For this review, take the finished solid that the model builds, in its own axes (mm). Give positions to 0.01 mm unless a question says otherwise; leave off trailing zeros. Write each loop counter-clockwise with the first axis right and the second up, starting at its lowest first coordinate (ties: lowest second). Pieces come first, ordered by that corner, then holes. Notation, with made-up numbers: M 47,-24.75 L 62,-24.75 A33 cw 62,10.25 Z; hole C -22,80 d11. An arc over 180 degrees is marked long. Use one line per item in the form item = value. Start each with the question number.
Q1. Consider section B-B on y = 0.5. Give the number of separate pieces and of enclosed holes in the cut face, and give its area (3 significant figures).
Q2. For probe 1 along X at (y, z) = (2.25, 0); probe 2 along Z at (x, y) = (5.09, 0.45); probe 3 along X at (y, z) = (2.55, -5.5), list the stretches that pass through material, from the lowest coordinate up. Write a range as [from, to].
Q3. Consider section A-A on x = 0.01. Write out the cut boundary in (y, z), and give its area (3 significant figures).
Q4. Clearance check with flat-ended pins moving along their axes: pin 1 Ø0.5 at (x, y) = (5.5, 2) entering from +Z; pin 2 Ø0.5 at (x, y) = (3, 2) entering from -Z; pin 3 Ø0.5 at (y, z) = (2, -4) entering from -X. State where each tip first meets the part, or that it passes through.
Q5. Consider section C-C on z = 4.5. Write out the cut boundary in (x, y), and give its area (3 significant figures).
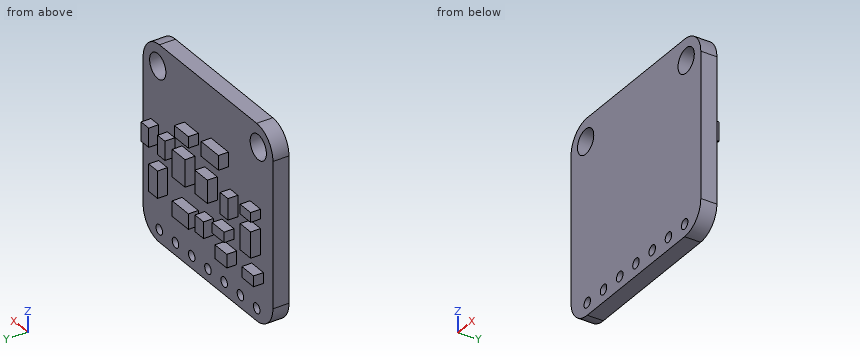
```python
from build123d import *

# Parameters (mm, degrees)
PCB_DEPTH          = 1.651
SKETCH2_R          = 1.27
SKETCH2_R_2        = 0.508
CUT_EXTRUDE1_DEPTH = 2.651
SKETCH3_W          = 1.9431
SKETCH3_H          = 2.3622
SKETCH3_W_2        = 2.0066
SKETCH3_H_2        = 2.794
SKETCH3_W_3        = 2.16822249
SKETCH3_H_3        = 1.167787324
SKETCH3_W_4        = 2.716171955
SKETCH3_H_4        = 1.493517176
SKETCH3_W_5        = 1.209663862
SKETCH3_H_5        = 2.17508788
SKETCH3_W_6        = 1.633321627
SKETCH3_H_6        = 2.659890245
SKETCH3_W_7        = 1.834361491
SKETCH3_H_7        = 1.100221283
SKETCH3_W_8        = 1.848311781
SKETCH3_H_8        = 1.38602823
SKETCH3_W_9        = 1.877433771
SKETCH3_H_9        = 1.066217503
SKETCH3_H_10       = 0.988618516
SKETCH3_W_10       = 1.152895283
SKETCH3_H_11       = 1.952725423
SKETCH3_W_11       = 1.201658639
SKETCH3_W_12       = 1.378437796
SKETCH3_H_12       = 2.778082819
SKETCH3_W_13       = 2.534678464
SKETCH3_H_13       = 1.568516227
SKETCH3_W_14       = 1.344087022
SKETCH3_H_14       = 1.688234225
COMPONENTS_DEPTH   = 1.016


with BuildPart() as part:
    # Sketch1 → pcb (new body)
    with BuildSketch(Plane(origin=(0, 0, 0), x_dir=(1, 0, 0), z_dir=(0, 1, 0))):
        with BuildLine():
            Line((-7.61, -10), (7.61, -10))
            ThreePointArc((7.61, -10), (9.406051224, -9.256051224), (10.15, -7.46))
            Line((10.15, -7.46), (10.15, 7.46))
            ThreePointArc((10.15, 7.46), (9.406051224, 9.256051224), (7.61, 10))
            Line((7.61, 10), (-7.61, 10))
            ThreePointArc((-7.61, 10), (-9.406051224, 9.256051224), (-10.15, 7.46))
            Line((-10.15, 7.46), (-10.15, -7.46))
            ThreePointArc((-10.15, -7.46), (-9.406051224, -9.256051224), (-7.61, -10))
        make_face()
    extrude(amount=PCB_DEPTH)

    # Sketch2 → Cut-Extrude1 (cut, through all)
    with BuildSketch(Plane.XZ):
        with Locations((-7.864, 7.714)):
            Circle(SKETCH2_R)
        with Locations((7.864, 7.714)):
            Circle(SKETCH2_R)
        with Locations((-7.61, -8.73)):
            Circle(SKETCH2_R_2)
        with Locations((-5.07, -8.73)):
            Circle(SKETCH2_R_2)
        with Locations((-2.53, -8.73)):
            Circle(SKETCH2_R_2)
        with Locations((0.01, -8.73)):
            Circle(SKETCH2_R_2)
        with Locations((2.55, -8.73)):
            Circle(SKETCH2_R_2)
        with Locations((5.09, -8.73)):
            Circle(SKETCH2_R_2)
        with Locations((7.63, -8.73)):
            Circle(SKETCH2_R_2)
    extrude(amount=-CUT_EXTRUDE1_DEPTH, mode=Mode.SUBTRACT)

    # Sketch3 → components (add)
    with BuildSketch(Plane(origin=(0, 1.651, 0), x_dir=(1, 0, 0), z_dir=(0, 1, 0))):
        with Locations((-0.47355, -0.1829)):
            Rectangle(SKETCH3_W, SKETCH3_H)
        with Locations((3.0507, -0.221)):
            Rectangle(SKETCH3_W_2, SKETCH3_H_2)
        with Locations((2.603432781, -3.639116092)):
            Rectangle(SKETCH3_W_3, SKETCH3_H_3)
        with Locations((-1.831635977, -4.030732119)):
            Rectangle(SKETCH3_W_4, SKETCH3_H_4)
        with Locations((-4.061190046, -0.08934394)):
            Rectangle(SKETCH3_W_5, SKETCH3_H_5)
        with Locations((-7.395465276, 1.673424229)):
            Rectangle(SKETCH3_W_6, SKETCH3_H_6)
        with Locations((-7.750024191, 5.108202568)):
            Rectangle(SKETCH3_W_7, SKETCH3_H_7)
        with Locations((-3.555135742, 5.251106041)):
            Rectangle(SKETCH3_W_8, SKETCH3_H_8)
        with Locations((-3.122473161, 3.062543074)):
            Rectangle(SKETCH3_W_9, SKETCH3_H_9)
        with Locations((-7.395465276, -1.123690742)):
            Rectangle(SKETCH3_W_6, SKETCH3_H_10)
        with Locations((5.77539067, -0.868377737)):
            Rectangle(SKETCH3_W_10, SKETCH3_H_11)
        with Locations((8.331105427, -0.868377737)):
            Rectangle(SKETCH3_W_11, SKETCH3_H_11)
        with Locations((7.041057209, 3.169050517)):
            Rectangle(SKETCH3_W_12, SKETCH3_H_12)
        with Locations((2.786660768, 4.379909938)):
            Rectangle(SKETCH3_W_13, SKETCH3_H_13)
        with Locations((-0.174043511, 4.013167629)):
            Rectangle(SKETCH3_W_14, SKETCH3_H_14)
    extrude(amount=COMPONENTS_DEPTH)


solid = part.part
```
Working result:
q1.separate_pieces = 1
q1.enclosed_holes = 9
q1.area = 385 mm²
q2.probe_1 = [-4.67, -3.46], [-1.45, 0.5], [2.05, 4.05], [5.2, 6.35], [7.73, 8.93]
q2.probe_2 = [-10, -9.24], [-8.22, 10]
q2.probe_3 = [-8.67, -6.83], [-4.48, -2.63]
q3.outline = M 0,-10 L 1.65,-10 L 1.65,-9.24 L 0,-9.24 Z; M 0,-8.22 L 1.65,-8.22 L 1.65,-4.86 L 2.67,-4.86 L 2.67,-3.17 L 1.65,-3.17 L 1.65,-1 L 2.67,-1 L 2.67,1.36 L 1.65,1.36 L 1.65,10 L 0,10 Z
q3.area = 35.5 mm²
q4.pin_1 = 1.84
q4.pin_2 = -5.16
q4.pin_3 = -0.85
q5.outline = M -10.15,0 L 10.15,0 L 10.15,1.65 L -0.47,1.65 L -0.47,2.67 L -3.19,2.67 L -3.19,1.65 L -10.15,1.65 Z
q5.area = 36.3 mm²
